For this review, take the finished solid that the model builds, in its own axes (mm). Face numbers are marked on the shaded views. A direction names the side the tool comes from. Give positions to 0.01 mm unless a question says otherwise; leave off trailing zeros. Write each loop counter-clockwise with the first axis right and the second up, starting at its lowest first coordinate (ties: lowest second). Pieces come first, ordered by that corner, then holes. Notation, with made-up numbers: M -14.75,58 L 0.25,58 A17 ccw 0.25,86 Z; hole C 62,-5.5 d10. An arc over 180 degrees is marked long. Write item = value, one per line.
```python
from build123d import *

# Parameters (mm, degrees)
SKETCH1_R            = 1.1375
SKETCH1_R_2          = 0.875
SKETCH1_R_3          = 1
BOSS_EXTRUDE1_DEPTH  = 9
CUT_EXTRUDE1_DEPTH   = 56.175080092
CUT_EXTRUDE2_REACH   = 58.746
SKETCH4_W            = 9.75
SKETCH4_H            = 6
CUT_EXTRUDE3_DEPTH   = 1.5
FILLET1_R            = 1
FILLET1_OF_MIRROR1_R = 1


with BuildPart() as part:
    # Sketch1 → Boss-Extrude1 (new body)
    with BuildSketch(Plane.XY):
        with BuildLine():
            Line((0, 0), (15.670430223, 0))
            Line((15.670430223, 0), (20.670430223, -5))
            ThreePointArc((20.670430223, -5), (24.313053668, -5), (24.313053668, -1.357376555))
            Line((24.313053668, -1.357376555), (16.71250591, 6.243171203))
            Line((16.71250591, 6.243171203), (16.71250591, 8.243171203))
            Line((16.71250591, 8.243171203), (50.666930898, 8.243171203))
            Line((50.666930898, 8.243171203), (50.666930898, 17.403556883))
            ThreePointArc((50.666930898, 17.403556883), (49.818924912, 19.279967227), (47.850198276, 19.883411807))
            Line((47.850198276, 19.883411807), (15.666930898, 15.772892856))
            ThreePointArc((15.666930898, 15.772892856), (12.366185788, 19.349870594), (7.521934274, 18.87773154))
            Line((7.521934274, 18.87773154), (3.918925439, 12.37773154))
            Line((3.918925439, 12.37773154), (-10.5, 8.243171203))
            Line((-10.5, 8.243171203), (-14, 8.243171203))
            Line((-14, 8.243171203), (-14, 0))
            Line((-14, 0), (-12.5, 0))
            Line((-12.5, 0), (-11.25, -2.25))
            Line((-11.25, -2.25), (-10, 0))
            Line((-10, 0), (-8.75, -2.25))
            Line((-8.75, -2.25), (-7.5, 0))
            Line((-7.5, 0), (-6.25, -2.25))
            Line((-6.25, -2.25), (-5, 0))
            Line((-5, 0), (-3.75, -2.25))
            Line((-3.75, -2.25), (-2.5, 0))
            Line((-2.5, 0), (-1.25, -2.25))
            Line((-1.25, -2.25), (0, 0))
        make_face()
        with Locations((10.418925439, 14.241576548)):
            Circle(SKETCH1_R, mode=Mode.SUBTRACT)
        with Locations((22.491741945, -3.178688277)):
            Circle(SKETCH1_R_2, mode=Mode.SUBTRACT)
        with Locations((48.166930898, 17.403556883)):
            Circle(SKETCH1_R_3, mode=Mode.SUBTRACT)
    extrude(amount=BOSS_EXTRUDE1_DEPTH)

    # Sketch3 → Cut-Extrude1 (cut, through all)
    with BuildSketch(Plane.XY.offset(9)):
        Polygon((-10.5, 1.35), (2, 1.35), (2, 8.35), align=None)
    extrude(amount=-CUT_EXTRUDE1_DEPTH, mode=Mode.SUBTRACT)

    # Cut-Extrude2: up to this plane
    cut_extrude2_end = Plane(origin=(2, 8.35, 0), z_dir=(-0.48860336893184564, 0.8725060159497188, 0))
    # Sketch4 → Cut-Extrude2 (cut, up to the surface)
    with BuildSketch(Plane(origin=(-2.981855105, 10.398964561, 0), x_dir=(0.9612616959383188, 0.2756373558169999, 0), z_dir=(-0.2756373558169999, 0.9612616959383188, 0)), mode=Mode.PRIVATE) as cut_extrude2_sk1:
        with Locations((-1.446121893, -4.5)):
            Rectangle(SKETCH4_W, SKETCH4_H)
    cut_extrude2_tool1 = split(extrude(cut_extrude2_sk1.sketch, amount=-CUT_EXTRUDE2_REACH, mode=Mode.PRIVATE), bisect_by=cut_extrude2_end, keep=Keep.BOTH, mode=Mode.PRIVATE)
    add(cut_extrude2_tool1.solids().sort_by_distance((-4.371957, 10.000359, 4.5))[0], mode=Mode.SUBTRACT)

    # Sketch5 → Cut-Extrude3 (cut)
    with BuildSketch(Plane.XY.offset(9)):
        with BuildLine():
            Line((16.200284742, 13.330448654), (44.30386483, 16.939697768))
            Line((44.30386483, 16.939697768), (45.056740957, 11.077394043))
            Line((45.056740957, 11.077394043), (16.200284742, 11.498637572))
            ThreePointArc((16.200284742, 11.498637572), (15.297651911, 12.414543113), (16.200284742, 13.330448654))
        make_face()
    cut_extrude3 = extrude(amount=-CUT_EXTRUDE3_DEPTH, mode=Mode.SUBTRACT)

    # Fillet1
    fillet1_edges = [part.edges().sort_by_distance(p)[0] for p in [
        (44.30386483, 16.939697768, 8.25),
        (45.056740957, 11.077394043, 8.25),
    ]]
    fillet(fillet1_edges, radius=FILLET1_R)

    # Mirror1: Cut-Extrude3 across plane
    add(cut_extrude3.mirror(Plane.XY.offset(4.5)), mode=Mode.SUBTRACT)

    # Fillet1 of Mirror1
    fillet1_of_mirror1_edges = [part.edges().sort_by_distance(p)[0] for p in [
        (44.30386483, 16.939697768, 0.75),
        (45.056740957, 11.077394043, 0.75),
    ]]
    fillet(fillet1_of_mirror1_edges, radius=FILLET1_OF_MIRROR1_R)


solid = part.part
```
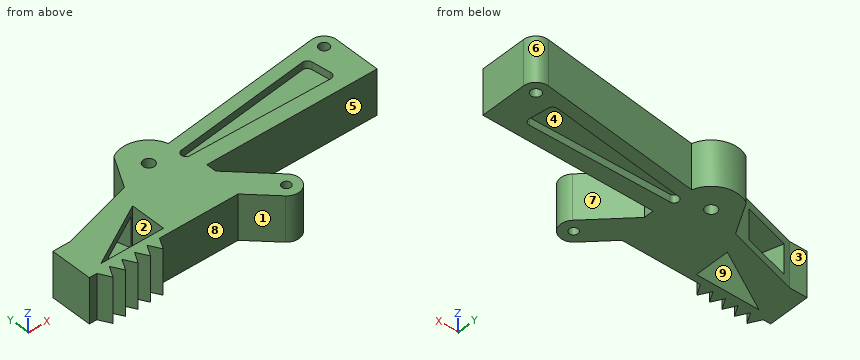
1. The part is to be moulded in two halves that separate along Y. For the marked faces 6, 7, 8 and 9, say which applies: +Y half, -Y half, draft (parallel to the pull), parting line (faces both ways), or undercut.
Responses:
face_6 = +Y half
face_7 = undercut
face_8 = -Y half
face_9 = undercut
2. We need section A-A, the plane x = 18.5. Write out the cut boundary in (y, z), then the cut area to 3 significant figures.
Responses:
outline = M -2.83,0 L 4.46,0 L 4.46,9 L -2.83,9 Z; M 8.24,0 L 11.47,0 L 11.47,1.5 L 13.63,1.5 L 13.63,0 L 16.13,0 L 16.13,9 L 13.63,9 L 13.63,7.5 L 11.47,7.5 L 11.47,9 L 8.24,9 Z
area = 130 mm2
3. We need section D-D, the plane x = 30. Write out the cut boundary in (y, z), then the cut area to 3 significant figures.
Responses:
outline = M 8.24,0 L 11.3,0 L 11.3,1.5 L 15.1,1.5 L 15.1,0 L 17.6,0 L 17.6,9 L 15.1,9 L 15.1,7.5 L 11.3,7.5 L 11.3,9 L 8.24,9 Z
area = 72.8 mm2
4. For line 1 along X through (y, z) = (-1.5, 5.25); line 2 along Y through (x, z) = (24, 1); line 3 along Y through (x, z) = (47.5, 7), list the stretches that pass through material, from the lowest coordinate up. Write a range as from..to.
Responses:
line_1 = -11.67..-10.83, -9.17..-8.33, -6.67..-5.83, -4.17..-3.33, -1.67..-0.83, 17.17..24.45
line_2 = -5.27..-1.04, 8.24..11.38, 14.33..16.84
line_3 = 8.24..16.66, 18.15..19.84
5. Machinability: for the marked faces 1, 2, 3, 4 and 5, which of the approach directions +Z, -Z, +X, -X, +Y, -Y give a long, thin tool a straight path to every point of the face, cutting with its end or side? Answer none if there is none.
Responses:
face_1 = +Z, -Z, -Y
face_2 = +Z, -Z
face_3 = +Z, -Z, -X, +Y
face_4 = -Z
face_5 = +Z, -Z, +X
6. We need section B-B, the plane x = 38.5. Write out the cut boundary in (y, z).
Responses:
outline = M 8.24,0 L 11.17,0 L 11.17,1.5 L 16.19,1.5 L 16.19,0 L 18.69,0 L 18.69,9 L 16.19,9 L 16.19,7.5 L 11.17,7.5 L 11.17,9 L 8.24,9 Z
7. Insertion check: P1, Ø2, axis at x = 32, z = 3.5, coming from the -Y side; P2, Ø4.5, axis at x = 7, z = 6, coming from the -Y side; P3, Ø0.6, axis at y = 7.5, z = 4, coming from the +X side; P4, Ø1.8, axis at x = 48.17, y = 17.4, coming from the -Z side. Each pin has a flat end and moves straight along its axis. Give the tip position at first contact, or say it passes through.
Responses:
P1 = 8.24
P2 = 0
P3 = 16.71
P4 = through
8. We need section C-C, the plane z = 3.75. Count the separate pieces of the cut face and the enclosed holes in it, then the cut area to 3 significant figures.
Responses:
separate_pieces = 1
enclosed_holes = 3
area = 705 mm2
